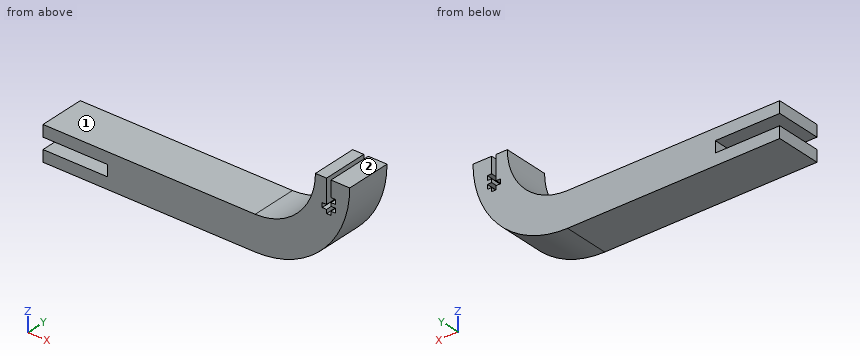
```python
from build123d import *

# Parameters (mm, degrees)
F1_DEPTH = 11


# Not quite as in the source:
# - ends of sketch curves that miss each other by under 0.0002 mm in the source are joined
# - a feature names something its author has since deleted; it is built from what else it names


with BuildPart() as f1:
    # F0 (on Front) → F1 (new body, symmetric)
    with BuildSketch(Plane.XZ):
        Polygon((-51.0195, -8.25), (51.0195, -8.25), (51.0195, 8.25), (-51.0195, 8.25), (-51.0195, 2.7), (-20.0195, 2.7), (-20.0195, -2.7), (-51.0195, -2.7), align=None)
        with BuildLine():
            Line((51.0195, 8.25), (51.0195, -8.25))
            ThreePointArc((51.0195, -8.25), (83.1651110764, 5.0651480786), (96.4802591551, 37.2107591551))
            Line((96.4802591551, 37.2107591551), (87.4802576721, 37.2107591551))
            Line((87.4802576721, 37.2107591551), (87.4802576721, 29.5374569684))
            Line((87.4802576721, 29.5374569684), (89.5802576721, 29.5374569684))
            Line((89.5802576721, 29.5374569684), (89.5802576721, 27.3874569684))
            Line((89.5802576721, 27.3874569684), (87.4802576721, 27.3874569684))
            Line((87.4802576721, 27.3874569684), (87.4802576721, 25.7107576162))
            Line((87.4802576721, 25.7107576162), (89.5802576721, 25.7107576162))
            Line((89.5802576721, 25.7107576162), (89.5802576721, 23.5607576162))
            Line((89.5802576721, 23.5607576162), (87.4802576721, 23.5607576162))
            Line((87.4802576721, 23.5607576162), (87.4802576721, 21.7607576162))
            Line((87.4802576721, 21.7607576162), (85.3302576721, 21.7607576162))
            Line((85.3302576721, 21.7607576162), (85.3302576721, 23.5607576162))
            Line((85.3302576721, 23.5607576162), (83.2302576721, 23.5607576162))
            Line((83.2302576721, 23.5607576162), (83.2302576721, 25.7107576162))
            Line((83.2302576721, 25.7107576162), (85.3302576721, 25.7107576162))
            Line((85.3302576721, 25.7107576162), (85.3302576721, 37.2107591551))
            Line((85.3302576721, 37.2107591551), (79.9802576721, 37.2107591551))
            ThreePointArc((79.9802576721, 37.2107591551), (71.4978497843, 16.7324093708), (51.0195, 8.25))
        make_face()
    extrude(amount=F1_DEPTH, both=True)


solid = f1.part
```
The model under review builds one solid part; all positions refer to its coordinate system, in mm. Face numbers are marked on the shaded views. A direction names the side the tool comes from. Give positions to 0.01 mm unless a question says otherwise; leave off trailing zeros. Write each loop counter-clockwise with the first axis right and the second up, starting at its lowest first coordinate (ties: lowest second). Pieces come first, ordered by that corner, then holes. Notation, with made-up numbers: M -32,69 L -5,69 A21 cw -5,87 Z; hole C 44,80 d11. An arc over 180 degrees is marked long. Write item = value, one per line. Start each with the question number.
Q1. For line 1 (Z direction, x = -25, y = 3.5); line 2 (Z direction, x = 38, y = 1.25); line 3 (X direction, y = -6.25, z = 30), list the stretches that pass through material, from the lowest coordinate up.
Q2. Clearance check with flat-ended pins moving along their axes: pin 1 (1.7 mm diameter, centred on x = 84.5, y = 2.5, fed in from -Z); pin 2 (1.1 mm diameter, centred on y = -0.5, z = 28.5, fed in from -X); pin 3 (1 mm diameter, centred on x = 48.5, y = -2.5, fed in from +Z). State where each tip first meets the part, or that it passes through.
Q3. We need section C-C (y = 6.75). State the section outline as (x, z) points.
Q4. We need section A-A (x = -26.5). State the section outline as (y, z) points.
Q5. We need section B-B (z = 34). State the section outline as (x, y) points, plus the area to 3 significant figures.
Q6. Machinability: for the marked faces 1 and 2, which of the approach directions +Z, -Z, +X, -X, +Y, -Y give a long, thin tool a straight path to every point of the face, cutting with its end or side? Answer none if there is none.
Q7. We need section D-D (x = 7.5). State the section outline as (y, z) points.
Result set:
q1.line_1 = -8.25 to -2.7, 2.7 to 8.25
q1.line_2 = -8.25 to 8.25
q1.line_3 = 79.07 to 85.33, 87.48 to 95.9
q2.pin_1 = 5.56
q2.pin_2 = 78.46
q2.pin_3 = 8.25
q3.outline = M -51.02,-8.25 L 51.02,-8.25 A45.46 ccw 96.48,37.21 L 87.48,37.21 L 87.48,29.54 L 89.58,29.54 L 89.58,27.39 L 87.48,27.39 L 87.48,25.71 L 89.58,25.71 L 89.58,23.56 L 87.48,23.56 L 87.48,21.76 L 85.33,21.76 L 85.33,23.56 L 83.23,23.56 L 83.23,25.71 L 85.33,25.71 L 85.33,37.21 L 79.98,37.21 A28.96 cw 51.02,8.25 L -51.02,8.25 L -51.02,2.7 L -20.02,2.7 L -20.02,-2.7 L -51.02,-2.7 Z
q4.outline = M -11,-8.25 L 11,-8.25 L 11,-2.7 L -11,-2.7 Z; M -11,2.7 L 11,2.7 L 11,8.25 L -11,8.25 Z
q5.outline = M 79.8,-11 L 85.33,-11 L 85.33,11 L 79.8,11 Z; M 87.48,-11 L 96.37,-11 L 96.37,11 L 87.48,11 Z
q5.area = 317 mm2
q6.face_1 = +Z, -X, +Y, -Y
q6.face_2 = +Z, +X, -X, +Y, -Y
q7.outline = M -11,-8.25 L 11,-8.25 L 11,8.25 L -11,8.25 Z
